Geometry check sheet. Reference: the model listing, model coordinates, mm. Round coordinates to 2 decimals unless told otherwise and drop trailing zeros. Write each loop counter-clockwise with the first axis right and the second up, starting at its lowest first coordinate (ties: lowest second). Pieces come first, ordered by that corner, then holes. Notation, with made-up numbers: M -16.5,53 L 42.5,53 A17 ccw 42.5,70 Z; hole C 32,33 d6. An arc over 180 degrees is marked long. One line per item, written item: value. Start each with the question number.
1. Depth check by flat-ended pin: P1, Ø3, axis at y = 137.5, z = 13, coming from the -X side; P2, Ø21.5, axis at x = 0, z = 0, coming from the +Y side; P3, Ø2, axis at y = 87, z = 9, coming from the -X side; P4, Ø8, axis at y = 22.5, z = -8.5, coming from the -X side. Enter the tip coordinate at first touch or a pass-through.
2. Scan lines: probe 1 along Y at (x, z) = (0, 18.7); probe 2 along X at (y, z) = (67, 0); probe 3 along X at (y, z) = (151, 2.5). Record each from-to range of solid material in increasing order. Write a range as [from, to].
3. Section check C-C (y = 172). Record the boundary of the cut face in (x, z), and give its area (3 significant figures).
4. Section check B-B (x = 6.5). Record the boundary of the cut face in (y, z).
5. Release check for a two-part mould opening along Z. For faces 1 (the cylindrical face through (5.407, 92.684, 17.169)), 2 (the flat face through (3, 188, -18)), 3 (the cylindrical face through (-19.524, 92.684, -4.336)) record: pulls with the +Z half, pulls with the -Z half, needs draft (parallel to the pull), parting line crosses it, or undercut.
6. Section check A-A (z = -12.5). Record the boundary of the cut face in (x, y).
from build123d import *

# Parameters (mm, degrees)
SKETCH_1_R                    = 20
EXTRUDE_1_DEPTH               = 188
CUT_EXTRUDE_2_DEPTH           = 191.115754213
CUT_EXTRUDE_2_DEPTH_BACK      = 191.115754213
SKETCH_2_R                    = 18
SKETCH_5_W                    = 1.45
SKETCH_5_H                    = 20
HOLE_WIZARD_M2_5_1_AT_2_COUNT = 2
HOLE_WIZARD_M2_5_1_AT_2_PITCH = 138


with BuildPart() as part:
    # 스케치1 → 보스-돌출1 (new body)
    with BuildSketch(Plane(origin=(0, 0, 0), x_dir=(1, 0, 0), z_dir=(0, 1, 0))):
        with Locations(Location((0, 0, 0), (0, 0, 270))):
            Circle(SKETCH_1_R)
    extrude(amount=EXTRUDE_1_DEPTH)

    # 스케치2 → 컷-돌출2 (cut, two sides: drawn at the far end of the back side and taken through both)
    with BuildSketch(Plane(origin=(0, 0, 0), x_dir=(1, 0, 0), z_dir=(0, 1, 0)).offset(-CUT_EXTRUDE_2_DEPTH_BACK)):
        with Locations(Location((0, 0, 0), (0, 0, 270))):
            Circle(SKETCH_2_R)
    extrude(amount=CUT_EXTRUDE_2_DEPTH + CUT_EXTRUDE_2_DEPTH_BACK, mode=Mode.SUBTRACT)

    # 스케치5 → M2.5 여유 구멍1 (revolve, cut)
    with BuildSketch(Plane(origin=(0, 163, 0), x_dir=(0, 1, 0), z_dir=(1, 0, 0))):
        with Locations((0.725, 10)):
            Rectangle(SKETCH_5_W, SKETCH_5_H)
    hole_wizard_m2_5_1 = revolve(axis=Axis((0, 163, -6.35), (0, 0, 1)), mode=Mode.SUBTRACT)

    # M2.5 여유 구멍1 at 2: M2.5 여유 구멍1 ×2
    with Locations(*[(0, -i * HOLE_WIZARD_M2_5_1_AT_2_PITCH, 0) for i in range(1, HOLE_WIZARD_M2_5_1_AT_2_COUNT)]):
        add(hole_wizard_m2_5_1, mode=Mode.SUBTRACT)


solid = part.part
Result sheet:
1. P1: stops at x = -16.36
1. P2: passes through
1. P3: stops at x = -18.33
1. P4: stops at x = -19.49
2. probe 1: y = [0, 23.55], [26.45, 161.55], [164.45, 188]
2. probe 2: x = [-20, -18], [18, 20]
2. probe 3: x = [-19.84, -17.83], [17.83, 19.84]
3. outline: C 0,0 d40; hole C 0,0 d36
3. area: 239 mm2
4. outline: M 0,-18.91 L 188,-18.91 L 188,-16.79 L 0,-16.79 Z; M 0,16.79 L 188,16.79 L 188,18.91 L 0,18.91 Z
5. face 1: undercut
5. face 2: needs draft
5. face 3: parting line crosses it
6. outline: M -15.61,0 L -12.95,0 L -12.95,188 L -15.61,188 Z; M 12.95,0 L 15.61,0 L 15.61,188 L 12.95,188 Z
